Design review of the part built by this model. Coordinates are the model's own, in mm. A direction names the side the tool comes from. Round coordinates to 2 decimals unless told otherwise and drop trailing zeros. Write each loop counter-clockwise with the first axis right and the second up, starting at its lowest first coordinate (ties: lowest second). Pieces come first, ordered by that corner, then holes. Notation, with made-up numbers: (-25.75, 46.25) -> (16.25, 46.25) arc R27 ccw to (16.25, 62.25) -> close; hole circle Ø7 at (29, 56.25). An arc over 180 degrees is marked (long way). Write item = value, one per line. Start each with the question number.
Item 1: For pin 1 Ø0.8 at (x, y) = (0, -3) entering from -Z; pin 2 Ø13 at (x, z) = (0, 0) entering from -Y; pin 3 Ø8 at (y, z) = (-18.5, 9) entering from +X, all flat-tipped, find the tip position at first contact; note any pin that passes through.
Item 2: Add section A-A, the plane x = 0. State the section outline as (y, z) points, then the cut area to 3 significant figures.
Item 3: Machinability: for faces 5 (the flat face through (-5, 4.5, 5)), 6 (the flat face through (0, -12, -10)), 7 (the flat face through (0, -12, 10)), 8 (the flat face through (0, -5, -2)), 9 (the flat face through (0, 4.4, -10)), which of the approach directions +Z, -Z, +X, -X, +Y, -Y give a long, thin tool a straight path to every point of the face, cutting with its end or side? Answer none if there is none.
Item 4: Mouldability with a two-part tool opening along Z and no side actions: class faces 1 (the cylindrical face through (-7.81, -15.14, 1.73)), 2 (the flat face through (0, -3, 2)), 3 (the flat face through (5, -25, -7)), 4 (the cylindrical face through (-10.75, -12.32, 0.18)) as released by +Z, released by -Z, zero draft, split by the parting line, or undercut.
Item 5: Add section D-D, the plane y = -15. State the section outline as (x, z) points, then the cut area to 3 significant figures.
Item 6: Add section C-C, the plane y = -4.25. State the section outline as (x, z) points, then the cut area to 3 significant figures.
Item 7: To check wall thickness, follow L1, parallel to X at y = 4.45, z = 0; L2, parallel to X at y = 0.4, z = 0; L3, parallel to X at y = -2.35, z = 0. State the ranges of each line that lie inside material, in increasing order.
Item 8: Add section B-B, the plane z = 0. State the section outline as (x, y) points, then the cut area to 3 significant figures.
from build123d import *

# Parameters (mm, degrees)
SKETCH_1_R            = 14
EXTRUDE_1_DEPTH       = 4.5
SKETCH_8_R            = 0.5
CUT_EXTRUDE_594_DEPTH = 0.1
CHAMFER_1_SIZE        = 2.5
SKETCH_2_R            = 10.75
EXTRUDE_2_DEPTH       = 25
CUT_EXTRUDE_START     = -25
CUT_EXTRUDE_1_DEPTH   = 25
SKETCH_4_R            = 6
CUT_EXTRUDE_2_DEPTH   = 5
CHAMFER_2_SIZE        = 0.5
SKETCH_6_R            = 8
CUT_EXTRUDE_3_DEPTH   = 20
CUT_EXTRUDE_4_DEPTH   = 32.5


with BuildPart() as part:
    # 草图1 → 凸台-拉伸1 (new body)
    with BuildSketch(Plane(origin=(0, 0, 0), x_dir=(1, 0, 0), z_dir=(0, 1, 0))):
        with Locations(Location((0, 0, 0), (0, 0, 270))):
            Circle(SKETCH_1_R)
    extrude(amount=EXTRUDE_1_DEPTH)

    # 草图8 → Cut-Extrude 594 (cut)
    with BuildSketch(Plane(origin=(0, 4.5, 0), x_dir=(1, 0, 0), z_dir=(0, 1, 0))):
        with Locations(Location((-10, 0, 0), (0, 0, 270))):
            Circle(SKETCH_8_R)
        with Locations(Location((0, 10, 0), (0, 0, 270))):
            Circle(SKETCH_8_R)
    extrude(amount=-CUT_EXTRUDE_594_DEPTH, mode=Mode.SUBTRACT)

    # 倒角1
    chamfer_1_edges = [part.edges().sort_by_distance(p)[0] for p in [
        (0, 4.5, -14),
    ]]
    chamfer(chamfer_1_edges, length=CHAMFER_1_SIZE)

    # 草图2 → 凸台-拉伸2 (add)
    with BuildSketch(Plane.XZ):
        with Locations(Location((0, 0, 0), (0, 0, 90))):
            Circle(SKETCH_2_R)
    extrude(amount=EXTRUDE_2_DEPTH)

    # 草图3 → 切除-拉伸1 (cut)
    with BuildSketch(Plane.XZ.offset(25).offset(CUT_EXTRUDE_START)):
        with BuildLine():
            Line((-3.94493346, -10), (3.94493346, -10))
            ThreePointArc((3.94493346, -10), (0, -10.75), (-3.94493346, -10))
        make_face()
        with BuildLine():
            Line((-3.94493346, 10), (3.94493346, 10))
            ThreePointArc((3.94493346, 10), (0, 10.75), (-3.94493346, 10))
        make_face()
    extrude(amount=CUT_EXTRUDE_1_DEPTH, mode=Mode.SUBTRACT)

    # 草图4 → 切除-拉伸2 (cut)
    with BuildSketch(Plane(origin=(0, 4.5, 0), x_dir=(1, 0, 0), z_dir=(0, 1, 0))):
        with Locations(Location((0, 0, 0), (0, 0, 270))):
            Circle(SKETCH_4_R)
    extrude(amount=-CUT_EXTRUDE_2_DEPTH, mode=Mode.SUBTRACT)

    # 倒角2
    chamfer_2_edges = [part.edges().sort_by_distance(p)[0] for p in [
        (0, 4.5, -6),
    ]]
    chamfer(chamfer_2_edges, length=CHAMFER_2_SIZE)

    # 草图6 → 切除-拉伸3 (cut)
    with BuildSketch(Plane.XZ.offset(25)):
        with Locations(Location((0, 0, 0), (0, 0, 270))):
            Circle(SKETCH_6_R)
    extrude(amount=-CUT_EXTRUDE_3_DEPTH, mode=Mode.SUBTRACT)

    # 草图7 → 切除-拉伸4 (cut, through all)
    with BuildSketch(Plane(origin=(0, -0.5, 0), x_dir=(1, 0, 0), z_dir=(0, 1, 0))):
        with BuildLine():
            Line((0.5, -2), (0.5, -1.414213562))
            ThreePointArc((0.5, -1.414213562), (0, 1.5), (-0.5, -1.414213562))
            Line((-0.5, -1.414213562), (-0.5, -2))
            Line((-0.5, -2), (0.5, -2))
        make_face()
    extrude(amount=-CUT_EXTRUDE_4_DEPTH, mode=Mode.SUBTRACT)


solid = part.part
Result set:
q1.pin_1 = -10
q1.pin_2 = -5
q1.pin_3 = 9.52
q2.outline = (-25, -10) -> (0, -10) -> (0, -14) -> (2, -14) -> (4.5, -11.5) -> (4.5, -10.5) -> (4.4, -10.5) -> (4.4, -9.5) -> (4.5, -9.5) -> (4.5, -6.5) -> (4, -6) -> (-0.5, -6) -> (-0.5, -1.5) -> (-5, -1.5) -> (-5, -8) -> (-25, -8) -> close; (-25, 8) -> (-5, 8) -> (-5, 2) -> (-0.5, 2) -> (-0.5, 6) -> (4, 6) -> (4.5, 6.5) -> (4.5, 11.5) -> (2, 14) -> (0, 14) -> (0, 10) -> (-25, 10) -> close
q2.area = 224 mm²
q3.face_5 = +Z, -Z, +X, -X, +Y
q3.face_6 = -Z, +X, -X, -Y
q3.face_7 = +Z, +X, -X, -Y
q3.face_8 = -Y
q3.face_9 = +Y
q4.face_1 = undercut
q4.face_2 = undercut
q4.face_3 = zero draft
q4.face_4 = split by the parting line
q5.outline = (-3.94, -10) -> (3.94, -10) arc R10.75 ccw to (3.94, 10) -> (-3.94, 10) arc R10.75 ccw to start; hole circle Ø16 at (0, 0)
q5.area = 154 mm²
q6.outline = (-3.94, -10) -> (3.94, -10) arc R10.75 ccw to (3.94, 10) -> (-3.94, 10) arc R10.75 ccw to start; hole (-0.5, 1.41) arc R1.5 ccw (long way) to (0.5, 1.41) -> (0.5, 2) -> (-0.5, 2) -> close
q6.area = 348 mm²
q7.L1 = -11.55 to -10.5, -9.5 to -6.45, 6.45 to 11.55
q7.L2 = -14 to -6, 6 to 14
q7.L3 = -10.75 to -1.5, 1.5 to 10.75
q8.outline = (-14, 0) -> (-10.75, 0) -> (-10.75, -25) -> (-8, -25) -> (-8, -5) -> (-1.5, -5) -> (-1.5, -0.5) -> (-6, -0.5) -> (-6, 4) -> (-6.5, 4.5) -> (-9.5, 4.5) -> (-9.5, 4.4) -> (-10.5, 4.4) -> (-10.5, 4.5) -> (-11.5, 4.5) -> (-14, 2) -> close; (1.5, -5) -> (8, -5) -> (8, -25) -> (10.75, -25) -> (10.75, 0) -> (14, 0) -> (14, 2) -> (11.5, 4.5) -> (6.5, 4.5) -> (6, 4) -> (6, -0.5) -> (1.5, -0.5) -> close
q8.area = 263 mm²
